```python
from build123d import *

# Parameters (mm, degrees)
SKETCH1_R           = 8.5
BOSS_EXTRUDE1_DEPTH = 10
SKETCH3_W           = 33.738328928
SKETCH3_H           = 8.707977782
BOSS_EXTRUDE2_DEPTH = 5


with BuildPart() as part:
    # Sketch1 → Boss-Extrude1 (new body)
    with BuildSketch(Plane(origin=(0, 0, 0), x_dir=(1, 0, 0), z_dir=(0, 1, 0))):
        with Locations(Location((0, 0, 0), (0, 0, 270))):
            Circle(SKETCH1_R)
    extrude(amount=BOSS_EXTRUDE1_DEPTH)

    # Sketch3 → Boss-Extrude2 (add)
    with BuildSketch(Plane.XZ):
        Rectangle(SKETCH3_W, SKETCH3_H)
    extrude(amount=-BOSS_EXTRUDE2_DEPTH)


solid = part.part
```
Check sheet for the modelled part. Datum: model origin and axes. Units: mm. A direction names the side the tool comes from. Coordinates: 2 decimals unless noted, no trailing zeros. Order: outer loops, then holes, each group sorted by start corner. A loop starts at its lowest first (then second) coordinate and runs counter-clockwise, first axis right, second up. Notation, with made-up numbers: M -11.75,58 L 46.25,58 A12 cw 46.25,71 Z; hole C 30.25,76 d9. An arc over 180 degrees is marked long. One line per question, with ' | ' between items. Start each with the question number.
Item 1: Sectioned sample at D-D on z = -6.25. Record the cut outline in (x, y).
Item 2: Access from +Z, -Z, +X, -X, +Y, -Y to the whole of each face (thin tool, end or side, straight path). Record for faces 1 (the flat face through (-12, 2, -4.354)), 2 (the cylindrical face through (8.428, 6.041, -1.107)), 3 (the flat face through (-12, 2, 4.354)), 4 (the flat face through (12, 2, 4.354)), 5 (the flat face through (12, 2, -4.354)).
Item 3: Sectioned sample at B-B on z = 0. Record the cut outline in (x, y), and give its area (3 significant figures).
Item 4: Gauge pin test, flat ends, axial feed: P1, Ø6, axis at x = -6, y = 5, coming from the -Z side; P2, Ø2.5, axis at x = 12, z = 1.5, coming from the +Y side; P3, Ø2, axis at y = 5.5, z = -6, coming from the -X side; P4, Ø1.5, axis at x = -9.5, z = -5.5, coming from the -Y side. Record the tip position at first contact, or that the pin passes through.
Item 5: Sectioned sample at C-C on x = -4.5. Record the cut outline in (y, z).
Item 6: Sectioned sample at A-A on y = 3.5. Record the cut outline in (x, z).
Item 7: Material ranges on line 1 (Z direction, x = 15.5, y = 2); line 2 (X direction, y = 5.25, z = -3); line 3 (X direction, y = 5.75, z = 3.5), recorded low to high.
Answer below:
1) outline: M -5.76,0 L 5.76,0 L 5.76,10 L -5.76,10 Z
2) face 1: -Z, -X, +Y, -Y | face 2: +Y | face 3: +Z, -X, +Y, -Y | face 4: +Z, +X, +Y, -Y | face 5: -Z, +X, +Y, -Y
3) outline: M -16.87,0 L 16.87,0 L 16.87,5 L 8.5,5 L 8.5,10 L -8.5,10 L -8.5,5 L -16.87,5 Z | area: 254 mm^2
4) P1: stops at z = -7.95 | P2: stops at y = 5 | P3: stops at x = -6.87 | P4: passes through
5) outline: M 0,-7.21 L 10,-7.21 L 10,7.21 L 0,7.21 Z
6) outline: M -16.87,-4.35 L -7.3,-4.35 A8.5 ccw 7.3,-4.35 L 16.87,-4.35 L 16.87,4.35 L 7.3,4.35 A8.5 ccw -7.3,4.35 L -16.87,4.35 Z
7) line 1: z = -4.35 to 4.35 | line 2: x = -7.95 to 7.95 | line 3: x = -7.75 to 7.75
